Could you check a few things on this model? Use its own coordinates, in mm. A direction names the side the tool comes from. Round coordinates to 2 decimals unless told otherwise and drop trailing zeros. Write each loop counter-clockwise with the first axis right and the second up, starting at its lowest first coordinate (ties: lowest second). Pieces come first, ordered by that corner, then holes. Notation, with made-up numbers: M -3,9 L 10,9 A8 cw 10,16 Z; hole C 82,-25.75 d7. An arc over 180 degrees is marked long. One line per item, written item: value. Start each with the question number.
(1) Which directions (+Z, -Z, +X, -X, +Y, -Y) give clear straight access to the entire face, cutting with the end or side of a thin tool? Please do faces 4 (the face through (-30.877, -36.331, -7.395)), 5 (the face through (32.479, 36.966, 61.619)), 6 (the face through (-33, -33, -15)), 7 (the face through (-38, -10, 35)).
(2) I want a section at B-B on z = 65.5. Please give me the cut outline in (x, y).
(3) I want a section at C-C on y = -15.5. Please give me the cut outline in (x, z).
(4) I'm going to push flat-ended pins straight in: pin 1 Ø5 at (x, y) = (33, 33) entering from +Z; pin 2 Ø6.5 at (x, y) = (-33, 33) entering from +Z; pin 3 Ø1 at (x, y) = (-32.5, 33.5) entering from +Z; pin 4 Ø12 at (x, y) = (7.5, -27) entering from -Z. Where does each tip first touch, or does it pass through?
(5) I want a section at A-A on x = 0. Please give me the cut outline in (y, z).
(6) Thinking about a two-plate mould opening in Y: for faces 1 (the face through (32.479, -29.034, 61.619)), 2 (the face through (-1, 41, 35)), 3 (the face through (36, 1, 70)), which applies, released by +Y, released by -Y, zero draft, split by the parting line, or undercut?
(7) I want a section at D-D on z = 9. Please give me the cut outline in (x, y), and give its area (3 significant figures).
(8) If I drill on L1, parallel to Y at x = 33, z = 64; L2, parallel to Z at x = 32.5, y = 21; L3, parallel to Y at x = 9, z = 63.5, over which ranges is the centre line in solid material (lowest first)?
```python
from build123d import *

# Parameters (mm, degrees)
SKETCH_1_W          = 82
SKETCH_1_H          = 82
SKETCH_1_R          = 35.5
EXTRUDE_1_DEPTH     = 70
SKETCH_4_R          = 4
CUT_EXTRUDE_2_DEPTH = 20
FILLET_2_R          = 3
FILLET_3_R          = 3
FILLET_4_R          = 3
FILLET_5_R          = 3
CUT_EXTRUDE_3_REACH = 92.896
SKETCH_3_W          = 8
SKETCH_3_H          = 20
SKETCH_5_R          = 3.95
EXTRUDE_2_DEPTH     = 15


with BuildPart() as part:
    # Sketch 1 → Extrude 1 (new body)
    with BuildSketch(Plane.XY):
        Rectangle(SKETCH_1_W, SKETCH_1_H)
        Circle(SKETCH_1_R, mode=Mode.SUBTRACT)
    extrude(amount=EXTRUDE_1_DEPTH)

    # Sketch 4 → Cut-Extrude 2 (cut)
    with BuildSketch(Plane.XY.offset(70)):
        with Locations((-33, 33)):
            Circle(SKETCH_4_R)
        with Locations((33, 33)):
            Circle(SKETCH_4_R)
        with Locations((33, -33)):
            Circle(SKETCH_4_R)
        with Locations((-33, -33)):
            Circle(SKETCH_4_R)
    extrude(amount=-CUT_EXTRUDE_2_DEPTH, mode=Mode.SUBTRACT)

    # Fillet 2
    fillet_2_edges = [part.edges().sort_by_distance(p)[0] for p in [
        (-37, 33, 50),
    ]]
    fillet(fillet_2_edges, radius=FILLET_2_R)

    # Fillet 3
    fillet_3_edges = [part.edges().sort_by_distance(p)[0] for p in [
        (29, 33, 50),
    ]]
    fillet(fillet_3_edges, radius=FILLET_3_R)

    # Fillet 4
    fillet_4_edges = [part.edges().sort_by_distance(p)[0] for p in [
        (-37, -33, 50),
    ]]
    fillet(fillet_4_edges, radius=FILLET_4_R)

    # Fillet 5
    fillet_5_edges = [part.edges().sort_by_distance(p)[0] for p in [
        (29, -33, 50),
    ]]
    fillet(fillet_5_edges, radius=FILLET_5_R)

    # Sketch 3 → Cut-Extrude 3 (cut, up to next)
    with BuildSketch(Plane.XY.offset(70), mode=Mode.PRIVATE) as cut_extrude_3_sk1:
        with Locations((-37, 0)):
            Rectangle(SKETCH_3_W, SKETCH_3_H)
    cut_extrude_3_tool1 = extrude(cut_extrude_3_sk1.sketch, amount=-CUT_EXTRUDE_3_REACH, mode=Mode.PRIVATE) & part.part
    add(cut_extrude_3_tool1.solids().sort_by_distance((-37, 0, 70))[0], mode=Mode.SUBTRACT)

    # Sketch 5 → Extrude 2 (add)
    with BuildSketch(Plane(origin=(0, 0, 0), x_dir=(-1, 0, 0), z_dir=(0, 0, -1))):
        with Locations((33, 33)):
            Circle(SKETCH_5_R)
        with Locations((-33, 33)):
            Circle(SKETCH_5_R)
        with Locations(Location((33, -33, 0), (0, 0, 180))):
            Circle(SKETCH_5_R)
        with Locations(Location((-33, -33, 0), (0, 0, 180))):
            Circle(SKETCH_5_R)
    extrude(amount=EXTRUDE_2_DEPTH)


solid = part.part
```
Found:
1. face 4: -Z
1. face 5: +Z
1. face 6: -Z, +X, -X, +Y, -Y
1. face 7: +Z, -Z, -X
2. outline: M -41,-41 L 41,-41 L 41,41 L -41,41 L -41,10 L -34.06,10 A35.5 cw long -34.06,-10 L -41,-10 Z; hole C -33,-33 d8; hole C -33,33 d8; hole C 33,-33 d8; hole C 33,33 d8
3. outline: M -41,0 L -31.94,0 L -31.94,70 L -41,70 Z; M 31.94,0 L 41,0 L 41,70 L 31.94,70 Z
4. pin 1: stops at z = 50.4
4. pin 2: stops at z = 51.02
4. pin 3: stops at z = 50.01
4. pin 4: passes through
5. outline: M -41,0 L -35.5,0 L -35.5,70 L -41,70 Z; M 35.5,0 L 41,0 L 41,70 L 35.5,70 Z
6. face 1: undercut
6. face 2: released by +Y
6. face 3: zero draft
7. outline: M -41,-41 L 41,-41 L 41,41 L -41,41 L -41,10 L -34.06,10 A35.5 cw long -34.06,-10 L -41,-10 Z
7. area: 2,650 mm²
8. L1: y = -41 to -37, -29 to -13.09, 13.09 to 29, 37 to 41
8. L2: z = 0 to 70
8. L3: y = -41 to -34.34, 34.34 to 41
